Design review of the part built by this model. Coordinates are the model's own, in mm. Face numbers are marked on the shaded views. A direction names the side the tool comes from. Coordinates: 2 decimals unless noted, no trailing zeros. Answer as a JSON object with one key per item and string values.
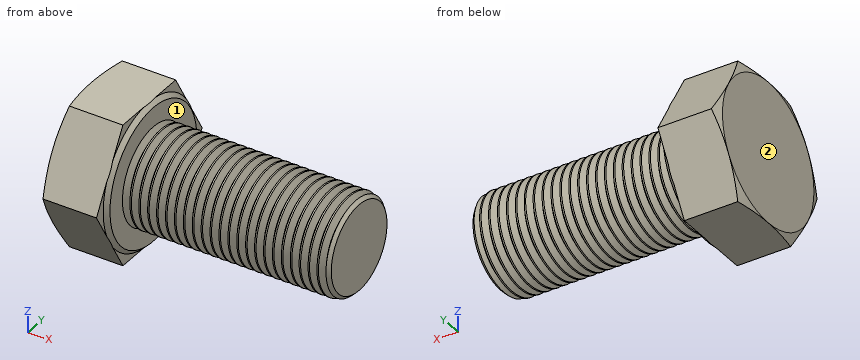
```python
from build123d import *

# Parameters (mm, degrees)
BASEHEAD_DEPTH   = 8.98
SKETCH5_R        = 7
BASEBODY_DEPTH   = 30
CHAMFER1_SIZE    = 0.7
LPATTERN10_COUNT = 23
LPATTERN10_PITCH = 1.299


with BuildPart() as part:
    # Sketch2 → BaseHead (new body)
    with BuildSketch(Plane(origin=(0, 0, 0), x_dir=(0, 0, -1), z_dir=(1, 0, 0))):
        Polygon((10.335, -5.966915032), (10.335, 5.966915032), (0, 11.933830064), (-10.335, 5.966915032), (-10.335, -5.966915032), (0, -11.933830064), align=None)
    extrude(amount=BASEHEAD_DEPTH)

    # Sketch3 → BearingFace (revolve, cut)
    with BuildSketch(Plane.XY, mode=Mode.PRIVATE) as bearingface_sk:
        Polygon((8.98, 11.933830064), (8.98, 9.82), (8.38, 10.42), (8.38, 11.933830064), align=None)
    revolve(bearingface_sk.sketch.rotate(Axis((-0.957090588, 0, 0), (1, 0, 0)), 90), axis=Axis((-0.957090588, 0, 0), (1, 0, 0)), mode=Mode.SUBTRACT)

    # Sketch4 → HeadChamfer (revolve, cut)
    with BuildSketch(Plane.XY):
        Polygon((0, 11.933830064), (0.581926553, 11.933830064), (0, 10.335), align=None)
    revolve(axis=Axis((-0.493528746, 0, 0), (1, 0, 0)), mode=Mode.SUBTRACT)

    # Sketch5 → BaseBody (add)
    with BuildSketch(Plane(origin=(8.98, 0, 0), x_dir=(0, 0, -1), z_dir=(1, 0, 0))):
        Circle(SKETCH5_R)
    extrude(amount=BASEBODY_DEPTH)

    # Chamfer1
    chamfer1_edges = [part.edges().sort_by_distance(p)[0] for p in [
        (38.98, 0, 7),
    ]]
    chamfer(chamfer1_edges, length=CHAMFER1_SIZE)

    # Sketch6 → Cut-Revolve10 (revolve, cut)
    with BuildSketch(Plane.XY, mode=Mode.PRIVATE) as cut_revolve10_sk:
        Polygon((8.98, 8.0825), (10.0625, 8.0825), (10.0625, 7), (9.52125, 6.0625275), (8.98, 7), align=None)
    cut_revolve10 = revolve(cut_revolve10_sk.sketch.rotate(Axis((-0.957090588, 0, 0), (1, 0, 0)), 90), axis=Axis((-0.957090588, 0, 0), (1, 0, 0)), mode=Mode.SUBTRACT)

    # LPattern10: Cut-Revolve10 ×23
    with Locations(*[(i * LPATTERN10_PITCH, 0, 0) for i in range(1, LPATTERN10_COUNT)]):
        add(cut_revolve10, mode=Mode.SUBTRACT)


solid = part.part
```
1) Wall thickness on probe 1 along X at (y, z) = (6.75, -7); probe 2 along Y at (x, z) = (15, -2.25); probe 3 along X at (y, z) = (9.5, 3.75): over which ranges is each line inside the solid? List them lowest first.
Completed:
{"probe 1": "0 to 8.98", "probe 2": "-6.15 to 6.15", "probe 3": "0 to 8.59"}
2) For the marked faces 1 and 2, list the 3-axis set-ups (+Z, -Z, +X, -X, +Y, -Y) from which the entire face can be reached by the end or side of a thin tool; tool diameter is ignored.
Completed:
{"face 1": "+X", "face 2": "+Z, -Z, -X, +Y, -Y"}
3) Clearance check with flat-ended pins moving along their axes: pin 1 Ø3 at (x, y) = (15.5, 5) entering from +Z; pin 2 Ø5 at (x, z) = (26.5, 7) entering from +Y; pin 3 Ø1.9 at (y, z) = (11, 2) entering from +X. State where each tip first meets the part, or that it passes through.
Completed:
{"pin 1": "z = 6.06", "pin 2": "y = 5.33", "pin 3": "x = 8.57"}
